Autodesk Inventor part; units mm, degrees
ref_plane "YZ Plane" through (0, 0, 0) normal (1, 0, 0) x (0, 1, 0)
ref_plane "XZ Plane" through (0, 0, 0) normal (0, 1, 0) x (-1, 0, 0)
ref_plane "XY Plane" through (0, 0, 0) normal (0, 0, 1) x (1, 0, 0)
sketch "Sketch1" plane through (0, 0, 0) normal (0, 1, 0) x (-1, 0, 0)
  line L0 (50, 50) -> (-50, 50)
  line L1 (-50, 50) -> (-50, -50)
  line L2 (-50, -50) -> (50, -50)
  line L3 (50, -50) -> (50, 50)
  line L4 (50, 50) -> (-50, -50) construction
  line L5 (-50, 50) -> (50, -50) construction
  point P0 (0, 0)
  dimension "d0" = 100
  dimension "d1" = 100
extrude "Extrusion1" add sketch "Sketch1" along normal blind 3
sketch "Sketch2" plane through (0, 3, 0) normal (0, 1, 0) x (1, 0, 0)
  circle A0 centre (-45, 45) radius 1.6
  line L0 (-50, 50) -> (-50, -50)
  line L1 (50, 50) -> (-50, 50)
  circle A1 centre (45, 45) radius 1.6
  circle A2 centre (45, -45) radius 1.6
  circle A3 centre (-45, -45) radius 1.6
  line L2 (50, -50) -> (50, 50)
  line L3 (-50, -50) -> (50, -50)
  point P0 (0, 0)
  dimension "d4" = 3.2
  dimension "d5" = 5
  dimension "d6" = 5
  dimension "d7" = 3.2
  dimension "d8" = 3.2
  dimension "d9" = 3.2
  dimension "d10" = 5
  dimension "d11" = 5
  dimension "d12" = 5
  dimension "d13" = 5
  dimension "d14" = 5
  dimension "d15" = 5
extrude "Extrusion2" cut sketch "Sketch2" against normal through all contours A0 | A1 | A2 | A3
properties part number "PCBV1" material "ABS Plastic"
Check sheet for the modelled part. Datum: model origin and axes. Units: mm. Coordinates: 2 decimals unless noted, no trailing zeros. Loops run counter-clockwise (first coordinate to the right, second up) from the corner with the lowest first, then second, coordinate; pieces in that order, holes last.
1) Gauge pin test, flat ends, axial feed: pin 1 (1 mm diameter, centred on x = 7, z = 12, fed in from -Y); pin 2 (1.9 mm diameter, centred on x = 45, z = -45, fed in from +Y). Record the tip position at first contact, or that the pin passes through.
2) Sectioned sample at A-A (x = -45). Record the boundary of the cut face in (y, z).
3) Material ranges on probe 1 along Z at (x, y) = (-45, 1.25), recorded low to high.
4) Sectioned sample at B-B (z = 45). Record the boundary of the cut face in (x, y).
5) Release check for a two-part mould opening along Z. For faces 1 (the face through (1, 1, -50)), 2 (the face through (-44.26, 1.52, 46.42)), 3 (the face through (45.74, 1.52, -43.58)), 4 (the face through (1, 0, 1)) record: released by +Z, released by -Z, zero draft, split by the parting line, or undercut.
Check sheet entries:
1. pin 1: stops at y = 0
1. pin 2: passes through
2. outline: (0, -50) - (3, -50) - (3, -46.6) - (0, -46.6) - close; (0, -43.4) - (3, -43.4) - (3, 43.4) - (0, 43.4) - close; (0, 46.6) - (3, 46.6) - (3, 50) - (0, 50) - close
3. probe 1: z = -50 to -46.6, -43.4 to 43.4, 46.6 to 50
4. outline: (-50, 0) - (-46.6, 0) - (-46.6, 3) - (-50, 3) - close; (-43.4, 0) - (43.4, 0) - (43.4, 3) - (-43.4, 3) - close; (46.6, 0) - (50, 0) - (50, 3) - (46.6, 3) - close
5. face 1: released by -Z
5. face 2: undercut
5. face 3: undercut
5. face 4: zero draft
